from build123d import *

# Parameters (mm, degrees)
F0_W          = 1219.2
F0_H          = 1219.2
F1_DEPTH      = 19.05
F2_W          = 1219.2
F2_H          = 1219.2
F2_W_2        = 1041.4
F2_H_2        = 476.25
F3_DEPTH      = 38.1
F4_W          = 101.6
F4_H          = 101.6
F5_DEPTH      = 914.4
F7_DEPTH      = 2867
F7_DEPTH_BACK = 1219.201


# Not quite as in the source:
# - an extrude ends at something that could not be found from the text; its depth is read off the source's solid


with BuildPart() as f1:
    # F0 (on Top) → F1 (new body)
    with BuildSketch(Plane.XY):
        with Locations((609.6, 609.6)):
            Rectangle(F0_W, F0_H)
    extrude(amount=F1_DEPTH)

    # F2 (on face) → F3 (join)
    with BuildSketch(Plane(origin=(0, 0, 0), x_dir=(1, 0, 0), z_dir=(0, 0, -1))):
        with Locations((609.6, -609.6)):
            Rectangle(F2_W, F2_H)
        with Locations((609.6, -892.175)):
            Rectangle(F2_W_2, F2_H_2, mode=Mode.SUBTRACT)
        with Locations((609.6, -327.025)):
            Rectangle(F2_W_2, F2_H_2, mode=Mode.SUBTRACT)
    extrude(amount=F3_DEPTH)

    # F4 (on face) → F5 (join)
    with BuildSketch(Plane.XY.offset(19.05)):
        with Locations((50.8, 1168.4)):
            Rectangle(F4_W, F4_H)
        with Locations((50.8, 50.8)):
            Rectangle(F4_W, F4_H)
        with Locations((1168.4, 50.8)):
            Rectangle(F4_W, F4_H)
        with Locations((1168.4, 1168.4)):
            Rectangle(F4_W, F4_H)
    extrude(amount=F5_DEPTH)

    # F6 (on face) → F7 (cut, two sides)
    with BuildSketch(Plane.XZ) as f7_sk:
        Polygon((0, 874.7912126503), (101.6, 933.45), (0, 933.45), align=None)
        Polygon((1219.2, 933.45), (1117.6, 933.45), (1219.2, 874.7912126503), align=None)
    extrude(amount=F7_DEPTH, mode=Mode.SUBTRACT)
    extrude(f7_sk.sketch, amount=-F7_DEPTH_BACK, mode=Mode.SUBTRACT)


solid = f1.part
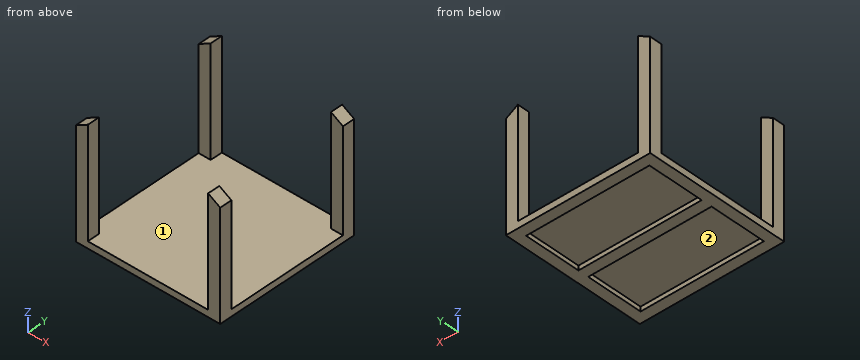
Source: CAD feature listing. Evaluate the final solid. Frame: model axes, mm. Face numbers are marked on the shaded views. Give positions to 0.01 mm unless a question says otherwise; leave off trailing zeros. Write each loop counter-clockwise with the first axis right and the second up, starting at its lowest first coordinate (ties: lowest second). Pieces come first, ordered by that corner, then holes. Notation, with made-up numbers: M 45,-25 L 78,-25 A20 cw 78,9 Z; hole C 58.5,-38.5 d5. An arc over 180 degrees is marked long. Return JSON: item names as keys, results as strings. Group by question number.
1) Draft query along Y for the marked faces 1 and 2. Return one class per face: released by +Y, released by -Y, zero draft, split by the parting line, or undercut.
2) Cut plane B-B, the plane x = 812.5. Output: boundary loops of the cut face in (y, z).
3) Ray query, L1, parallel to X at y = 1151, z = 603.5; L2, parallel to Z at x = 51, y = 863.5; L3, parallel to Z at x = 1057, y = 330.5. Return the intervals inside material, ascending.
4) First-contact query: pin 1 Ø3 at (x, y) = (304.5, 142) entering from +Z. Flat tip, straight axial feed; report the tip coordinate or a pass-through.
5) Cut plane A-A, the plane z = 628. Output: boundary loops of the cut face in (x, y), then the cut area to 3 significant figures.
6) Cut plane C-C, the plane y = 802. Output: boundary loops of the cut face in (x, z).
Data:
{
 "1": {"face 1": "undercut", "face 2": "undercut"},
 "2": {"outline": "M 0,-38.1 L 88.9,-38.1 L 88.9,0 L 565.15,0 L 565.15,-38.1 L 654.05,-38.1 L 654.05,0 L 1130.3,0 L 1130.3,-38.1 L 1219.2,-38.1 L 1219.2,19.05 L 0,19.05 Z"},
 "3": {"L1": "x = 0 to 101.6, 1117.6 to 1219.2", "L2": "z = -38.1 to 19.05", "L3": "z = 0 to 19.05"},
 "4": {"pin 1": "stops at z = 19.05"},
 "5": {"outline": "M 0,0 L 101.6,0 L 101.6,101.6 L 0,101.6 Z; M 0,1117.6 L 101.6,1117.6 L 101.6,1219.2 L 0,1219.2 Z; M 1117.6,0 L 1219.2,0 L 1219.2,101.6 L 1117.6,101.6 Z; M 1117.6,1117.6 L 1219.2,1117.6 L 1219.2,1219.2 L 1117.6,1219.2 Z", "area": "41,300 mm²"},
 "6": {"outline": "M 0,-38.1 L 88.9,-38.1 L 88.9,0 L 1130.3,0 L 1130.3,-38.1 L 1219.2,-38.1 L 1219.2,19.05 L 0,19.05 Z"}
}
